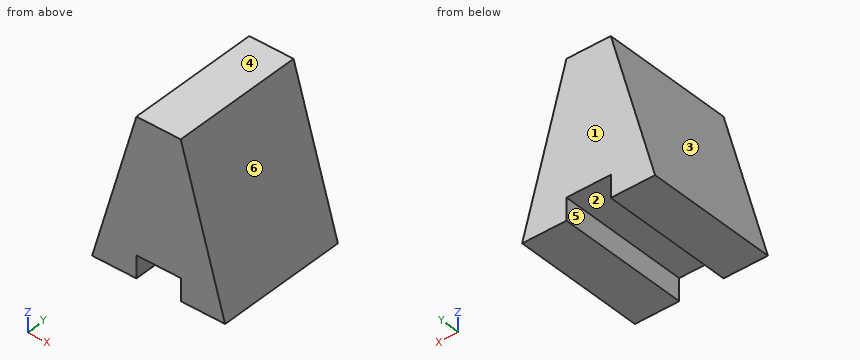
from build123d import *

# Parameters (mm, degrees)
F0_W     = 38.1
F0_H     = 44.45
F1_DEPTH = 38.1
F2_W     = 12.7
F2_H     = 6.35
F3_DEPTH = 65.532
F5_DEPTH = 60.706
F7_DEPTH = 60.706


with BuildPart() as f1:
    # F0 (on Front) → F1 (new body)
    with BuildSketch(Plane.XZ):
        with Locations((19.05, 22.225)):
            Rectangle(F0_W, F0_H)
    extrude(amount=F1_DEPTH)

    # F2 (on face) → F3 (cut)
    with BuildSketch(Plane.XZ.offset(38.1)):
        with Locations((19.05, 3.175)):
            Rectangle(F2_W, F2_H)
    extrude(amount=-F3_DEPTH, mode=Mode.SUBTRACT)

    # F4 (on face) → F5 (cut)
    with BuildSketch(Plane.XZ.offset(38.1)):
        Polygon((0, 0), (12.7, 44.45), (0, 44.45), align=None)
    extrude(amount=-F5_DEPTH, mode=Mode.SUBTRACT)

    # F6 (on face) → F7 (cut)
    with BuildSketch(Plane.XZ.offset(38.1)):
        Polygon((38.1, 44.45), (25.4, 44.45), (38.1, 0), align=None)
    extrude(amount=-F7_DEPTH, mode=Mode.SUBTRACT)


solid = f1.part
Input: part model. Units: mm. Frame: model coordinates. Face numbers are marked on the shaded views. A direction names the side the tool comes from. Give positions to 0.01 mm unless a question says otherwise; leave off trailing zeros. Loops run counter-clockwise (first coordinate to the right, second up) from the corner with the lowest first, then second, coordinate; pieces in that order, holes last. Notation, with made-up numbers: (25, 86.5) - (72, 86.5) arc R29 cw to (72, 117.5) - close; hole circle Ø8 at (3, 8.25). An arc over 180 degrees is marked (long way). Use CSV: the item, a comma, the result in double quotes. Start each with the question number.
Item 1: Section D-D on z = 28. Return loops of the section in (x, y), then the cut area to 3 significant figures.
Item 2: Section C-C on x = 8.5. Return loops of the section in (y, z), then the cut area to 3 significant figures.
Item 3: Section A-A on z = 3.5. Return loops of the section in (x, y), then the cut area to 3 significant figures.
Item 4: Reachability of the marked faces 1 and 2 from +Z, -Z, +X, -X, +Y, -Y: full face, straight path, thin tool, end or side. Return the list, or none.
Item 5: Section B-B on y = -10. Return loops of the section in (x, z), then the cut area to 3 significant figures.
Item 6: Line query: line 1 (Z direction, x = 25, y = -24); line 2 (X direction, y = -29, z = 16); line 3 (X direction, y = -12, z = 20.5). Output: solid intervals per line, ascending.
Item 7: Contact query for flat-ended pins moving along their axis: P1, Ø5, axis at y = -7, z = 14.5, coming from the -X side; P2, Ø8, axis at x = 20, y = -16.5, coming from the -Z side; P3, Ø3, axis at y = -21.5, z = 4, coming from the +X side. Output: stop coordinate, or through.
Item 8: Mould query, pull axis X, two halves, no side actions, for the marked faces 3, 4, 5 and 6. Classes: pulls with the +X half, pulls with the -X half, needs draft (parallel to the pull), parting line crosses it, or undercut.
Ans:
1,outline,"(8, -38.1) - (30.1, -38.1) - (30.1, 0) - (8, 0) - close"
1,area,"842 mm2"
2,outline,"(-38.1, 0) - (0, 0) - (0, 29.75) - (-38.1, 29.75) - close"
2,area,"1,130 mm2"
3,outline,"(1, -38.1) - (12.7, -38.1) - (12.7, 0) - (1, 0) - close; (25.4, -38.1) - (37.1, -38.1) - (37.1, 0) - (25.4, 0) - close"
3,area,"892 mm2"
4,face 1,"+Z, -Z, +X, -X, +Y"
4,face 2,"-Z, +Y, -Y"
5,outline,"(0, 0) - (12.7, 0) - (12.7, 6.35) - (25.4, 6.35) - (25.4, 0) - (38.1, 0) - (25.4, 44.45) - (12.7, 44.45) - close"
5,area,"1,050 mm2"
6,line 1,"z = 6.35 to 44.45"
6,line 2,"x = 4.57 to 33.53"
6,line 3,"x = 5.86 to 32.24"
7,P1,"stops at x = 3.43"
7,P2,"stops at z = 6.35"
7,P3,"stops at x = 37.39"
8,face 3,"pulls with the -X half"
8,face 4,"needs draft"
8,face 5,"undercut"
8,face 6,"pulls with the +X half"
